from build123d import *

# Parameters (mm, degrees)
F0_W      = 50
F0_H      = 150
F0_H_2    = 50
F0_W_2    = 70
F0_H_3    = 40
F1_DEPTH  = 10
F2_R      = 3.175
F3_DEPTH  = 10.001
F4_R      = 5.5
F5_DEPTH  = 10.001
F6_R      = 5.5
F7_DEPTH  = 10.001
F9_DEPTH  = 10.001
F11_D     = 2
F13_D     = 2
F14_R     = 5.5
F14_R_2   = 2.7
F15_DEPTH = 4
F16_DEPTH = 4


# Not quite as in the source:
# - a pattern or mirror of a feature is missing from the dataset's text; its kind, count and spacing are read off the source's solid
# - a feature names something its author has since deleted; it is built from what else it names


with BuildPart() as f1:
    # F0 (on Top) → F1 (new body)
    with BuildSketch(Plane.XY):
        Rectangle(F0_W, F0_H)
        with Locations((0, 100)):
            Rectangle(F0_W, F0_H_2)
        with Locations((60, 100)):
            Rectangle(F0_W_2, F0_H_2)
        with Locations((-60, 100)):
            Rectangle(F0_W_2, F0_H_2)
        with Locations((0, -100)):
            Rectangle(F0_W, F0_H_2)
        with Locations((60, -100)):
            Rectangle(F0_W_2, F0_H_2)
        with Locations((0, 145)):
            Rectangle(F0_W, F0_H_3)
        with Locations((-60, -100)):
            Rectangle(F0_W_2, F0_H_2)
    extrude(amount=F1_DEPTH)

    # F2 (on face) → F3 (cut, through all)
    with BuildSketch(Plane.XY.offset(10)):
        with Locations((0, 157.825)):
            Circle(F2_R)
    extrude(amount=-F3_DEPTH, mode=Mode.SUBTRACT)

    # F4 (on face) → F5 (cut, through all)
    with BuildSketch(Plane.XY.offset(10)):
        with Locations((-84.5, 100)):
            Circle(F4_R)
    extrude(amount=-F5_DEPTH, mode=Mode.SUBTRACT)

    # F6 (on face) → F7 (cut, through all)
    with BuildSketch(Plane.XY.offset(10)):
        with Locations((84.5, 100)):
            Circle(F6_R)
    extrude(amount=-F7_DEPTH, mode=Mode.SUBTRACT)

    # F8 (on face) → F9 (cut, through all)
    with BuildSketch(Plane.XY.offset(10)):
        with BuildLine():
            Line((73.023525645, 81.2305957373), (84.5, 85))
            ThreePointArc((84.5, 85), (69.5, 100), (84.5, 115))
            Line((84.5, 115), (73.5817295179, 119.0995122891))
            ThreePointArc((73.5817295179, 119.0995122891), (62.5023896916, 100.3242540951), (73.023525645, 81.2305957373))
        make_face()
        with BuildLine():
            Line((-84.5, 85), (-73.023525645, 81.2305957373))
            ThreePointArc((-73.023525645, 81.2305957373), (-62.5023896916, 100.3242540951), (-73.5817295179, 119.0995122891))
            Line((-73.5817295179, 119.0995122891), (-84.5, 115))
            ThreePointArc((-84.5, 115), (-69.5, 100), (-84.5, 85))
        make_face()
    extrude(amount=-F9_DEPTH, mode=Mode.SUBTRACT)

    # F11 (through all)
    with Locations(Plane.XY.offset(10)):
        with Locations((88, -82), (88, -118)):
            f11 = Hole(F11_D / 2)

    # F11_copies: F11 across plane
    add(f11.mirror(Plane(origin=(0, 0, 0), x_dir=(0, 0, -1), z_dir=(-1, 0, 0))), mode=Mode.SUBTRACT)

    # F13 (through all)
    with Locations(Plane(origin=(0, 0, 0), x_dir=(1, 0, 0), z_dir=(0, 0, -1))):
        with Locations((17.5, -21), (17.5, 9)):
            Hole(F13_D / 2)

    # F14 (on Top) → F15 (join)
    with BuildSketch(Plane.XY):
        with Locations((84.5, 100)):
            Circle(F14_R)
        with Locations((84.5, 100)):
            Circle(F14_R_2, mode=Mode.SUBTRACT)
        with Locations((-84.5, 100)):
            Circle(F14_R)
        with Locations((-84.5, 100)):
            Circle(F14_R_2, mode=Mode.SUBTRACT)
    extrude(amount=F15_DEPTH)

    # F14 (on Top) → F16 (join)
    with BuildSketch(Plane.XY):
        with Locations((84.5, 100)):
            Circle(F14_R)
        with Locations((84.5, 100)):
            Circle(F14_R_2, mode=Mode.SUBTRACT)
        with Locations((-84.5, 100)):
            Circle(F14_R)
        with Locations((-84.5, 100)):
            Circle(F14_R_2, mode=Mode.SUBTRACT)
    extrude(amount=F16_DEPTH)


solid = f1.part
Geometry check sheet. Reference: the model listing, model coordinates, mm. A direction names the side the tool comes from. Give positions to 0.01 mm unless a question says otherwise; leave off trailing zeros. Write each loop counter-clockwise with the first axis right and the second up, starting at its lowest first coordinate (ties: lowest second). Pieces come first, ordered by that corner, then holes. Notation, with made-up numbers: M 42.5,12.25 L 53.5,12.25 A33 cw 53.5,44.25 Z; hole C 77,55.25 d11. An arc over 180 degrees is marked long. One line per question, with ' | ' between items.
1. Gauge pin test, flat ends, axial feed: pin 1 (1.8 mm diameter, centred on x = -88, y = -118, fed in from -Z); pin 2 (5 mm diameter, centred on x = -55, z = 3, fed in from +Y); pin 3 (5 mm diameter, centred on y = -65.5, z = 4, fed in from -X); pin 4 (8.5 mm diameter, centred on x = 84.5, y = 100, fed in from +Z). Record the tip position at first contact, or that the pin passes through.
Ans:
pin 1: through | pin 2: y = 125 | pin 3: x = -25 | pin 4: z = 4
2. Scan lines: line 1 along Y through (x, z) = (-88, 2); line 2 along Y through (x, z) = (17.5, 6.75); line 3 along Y through (x, z) = (59.5, 3.25). Record each from-to range of solid material in increasing order. Write a range as from..to.
Ans:
line 1: -125..-119, -117..-83, -81..-75, 75..125 | line 2: -125..-10, -8..20, 22..165 | line 3: -125..-75, 75..125
3. Cross-section at B-B (y = -60.5). Enter the section's corners in (x, z), plus the area to 3 significant figures.
Ans:
outline: M -25,0 L 25,0 L 25,10 L -25,10 Z | area: 500 mm2
4. Cross-section at A-A (x = -57.5). Enter the section's corners in (y, z), plus the area to 3 significant figures.
Ans:
outline: M -125,0 L -75,0 L -75,10 L -125,10 Z; M 75,0 L 125,0 L 125,10 L 75,10 Z | area: 1,000 mm2
5. Mould release check, pull along X, two halves, no side actions. Record for faces 1 (the face through (60, -75, 5)), 2 (the face through (-78.96, 117.08, 5.07)), 3 (the face through (25, -1, 5)): released by +X, released by -X, zero draft, split by the parting line, or undercut.
Ans:
face 1: zero draft | face 2: undercut | face 3: released by +X
6. Set-up check for faces 4 (the face through (-60, 125, 5)), 5 (the face through (62.51, 100.64, 5.07)), 6 (the face through (95, 100, 5)), 7 (the face through (-88.55, 103.72, 7.04)): record each of +Z, -Z, +X, -X, +Y, -Y from which the full face is reachable in a straight line by a thin tool's end or side.
Ans:
face 4: +Z, -Z, -X, +Y | face 5: +Z, -Z | face 6: +Z, -Z, +X, +Y, -Y | face 7: +Z
